Geometry: see drawing. Coordinates: mm, zero at the bounding-box minimum. Give positions to 0.01 mm unless a question says otherwise; leave off trailing zeros. Order: outer loops, then holes, each group sorted by start corner. A loop starts at its lowest first (then second) coordinate and runs counter-clockwise, first axis right, second up. Notation, with made-up numbers: (-26.75, 51) - (28.25, 51) arc R15 ccw to (28.25, 78) - close; hole circle Ø3 at (13, -38). An arc over 180 degrees is marked (long way). One line per item, written item: value.
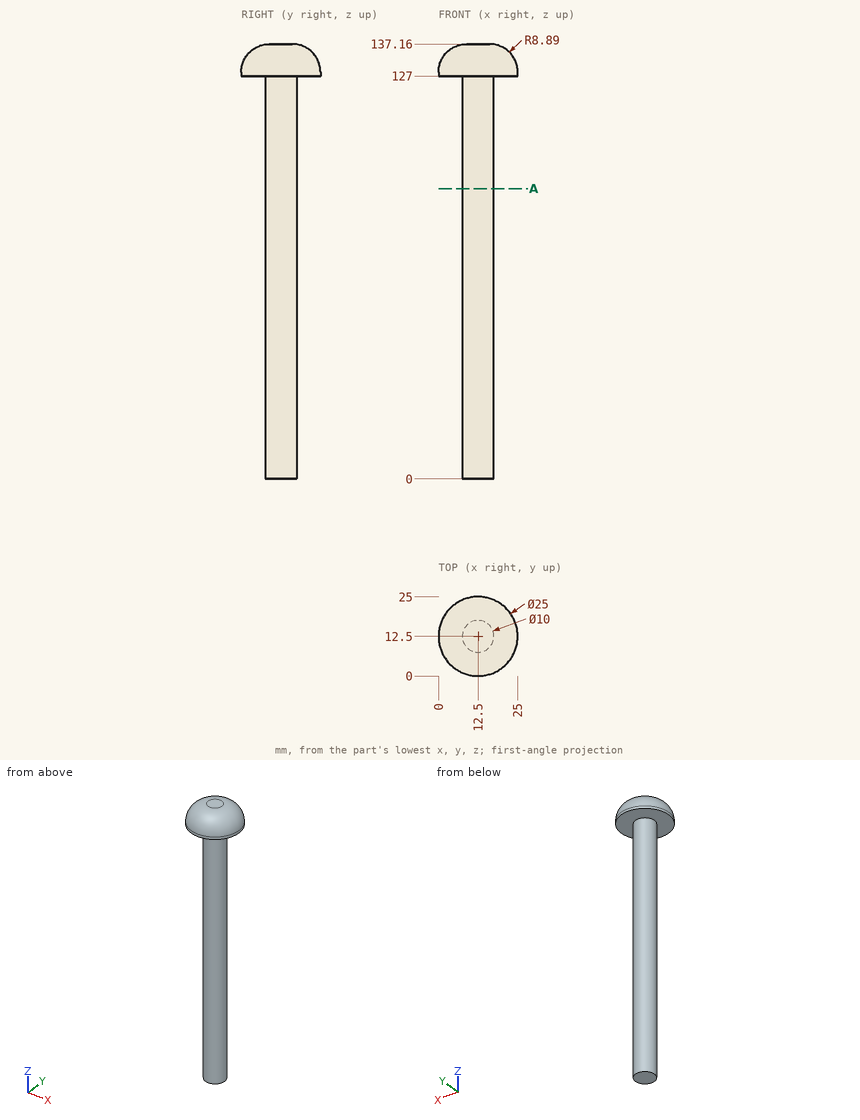
1) First-contact query: pin 1 (4 mm diameter, centred on x = 12.5, z = 68, fed in from +Y); pin 2 (2 mm diameter, centred on x = 19, y = 3.5, fed in from -Z); pin 3 (1.5 mm diameter, centred on x = 14, y = 20.5, fed in from +Z). Flat tips, straight axial feed; report the tip coordinate or a pass-through.
Answers below:
pin 1: y = 17.5
pin 2: z = 127
pin 3: z = 136.32
2) Material intervals for line 1 along Y through (x, z) = (12, 80); line 2 along X through (y, z) = (12.25, 27.5); line 3 along X through (y, z) = (11, 60), sorted ascending.
Answers below:
line 1: 7.53 to 17.47
line 2: 7.51 to 17.49
line 3: 7.73 to 17.27
3) Section A-A, the plane z = 91.5. Return loops of the section in (x, y), then the cut area to 3 significant figures.
Answers below:
outline: circle Ø10 at (12.5, 12.5)
area: 78.5 mm^2
